```python
from build123d import *

# Parameters (mm, degrees)
SKETCH1_R           = 17.1
BOSS_EXTRUDE1_DEPTH = 59.5
SKETCH2_R           = 4.75
BOSS_EXTRUDE2_DEPTH = 2
FILLET1_R           = 0.635
FILLET2_R           = 0.635


with BuildPart() as part:
    # Sketch1 → Boss-Extrude1 (new body)
    with BuildSketch(Plane.XY):
        with Locations(Location((0, 0, 0), (0, 0, 180))):
            Circle(SKETCH1_R)
    extrude(amount=BOSS_EXTRUDE1_DEPTH)

    # Sketch2 → Boss-Extrude2 (add)
    with BuildSketch(Plane.XY.offset(59.5)):
        Circle(SKETCH2_R)
    extrude(amount=BOSS_EXTRUDE2_DEPTH)

    # Fillet1
    fillet1_edges = [part.edges().sort_by_distance(p)[0] for p in [
        (17.1, 0, 59.5),
        (-4.75, 0, 61.5),
    ]]
    fillet(fillet1_edges, radius=FILLET1_R)

    # Fillet2
    fillet2_edges = [part.edges().sort_by_distance(p)[0] for p in [
        (17.1, 0, 0),
    ]]
    fillet(fillet2_edges, radius=FILLET2_R)


solid = part.part
```
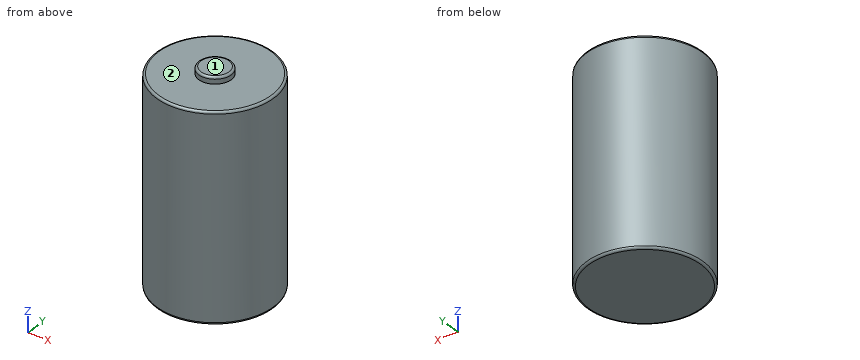
The listing builds one solid part. Answer for the finished solid, in the listing's coordinates (mm). Face numbers are marked on the shaded views. A direction names the side the tool comes from. Round coordinates to 2 decimals unless told otherwise and drop trailing zeros. Write each loop counter-clockwise with the first axis right and the second up, starting at its lowest first coordinate (ties: lowest second). Pieces come first, ordered by that corner, then holes. Notation, with made-up numbers: (18, 77) -> (73, 77) arc R24 ccw to (73, 110) -> close; hole circle Ø10 at (63.25, 15). An arc over 180 degrees is marked (long way). Answer as a JSON object with one key per item and string values. Group by question number.
Q1. Section A-A (x = 0) is taken. Write down the section's boundary in (y, z) (3 decimals), plus the area to 3 significant figures.
Q2. Straight lines are drawn through the part: line 1 along Y through (x, z) = (0.5, 10.5); line 2 along Z through (x, y) = (14, -0.5); line 3 along Y through (x, z) = (14, 19). For each, find the intervals that lie inside material, in ascending order.
Q3. Each of these flat-tipped pins is pushed along its axis until it touches: pin 1 Ø1 at (y, z) = (-9, 44) entering from +X; pin 2 Ø4 at (y, z) = (-7.5, 42.5) entering from +X; pin 3 Ø8 at (x, y) = (3, 9) entering from +Z. Where does it stop, or does it pass through?
Q4. Section C-C (z = 46.5) is taken. Write down the section's boundary in (x, y).
Q5. Which of the six approach directions +Z, -Z, +X, -X, +Y, -Y give full straight-line access (tool end or side, diameter ignored) to the marked faces 1 and 2?
Check values:
{
 "1": {"outline": "(-17.1, 0.635) arc R0.635 ccw to (-16.465, 0) -> (16.465, 0) arc R0.635 ccw to (17.1, 0.635) -> (17.1, 58.865) arc R0.635 ccw to (16.465, 59.5) -> (4.75, 59.5) -> (4.75, 60.865) arc R0.635 ccw to (4.115, 61.5) -> (-4.115, 61.5) arc R0.635 ccw to (-4.75, 60.865) -> (-4.75, 59.5) -> (-16.465, 59.5) arc R0.635 ccw to (-17.1, 58.865) -> close", "area": "2,050 mm^2"},
 "2": {"line 1": "-17.09 to 17.09", "line 2": "0 to 59.5", "line 3": "-9.82 to 9.82"},
 "3": {"pin 1": "x = 14.84", "pin 2": "x = 16.19", "pin 3": "z = 59.5"},
 "4": {"outline": "circle Ø34.2 at (0, 0)"},
 "5": {"face 1": "+Z, +X, -X, +Y, -Y", "face 2": "+Z"}
}
